Could you check a few things on this model? Use its own coordinates, in mm. Face numbers are marked on the shaded views. Round coordinates to 2 decimals unless told otherwise and drop trailing zeros. Order: outer loops, then holes, each group sorted by start corner. A loop starts at its lowest first (then second) coordinate and runs counter-clockwise, first axis right, second up.
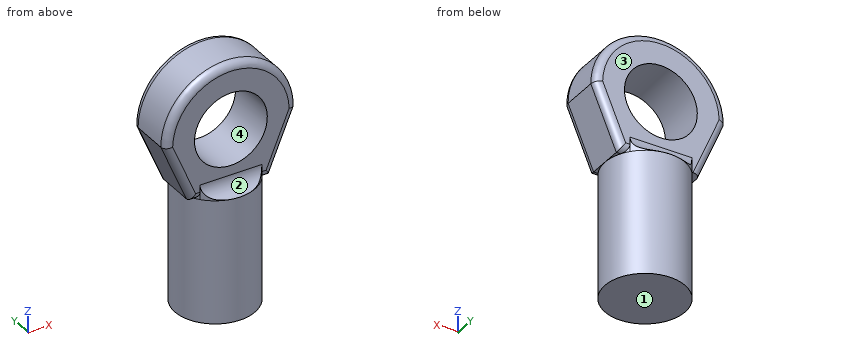
```python
from build123d import *

# Parameters (mm, degrees)
EXTRUDE_1_DEPTH     = 3.5
SKETCH_2_R          = 2.75
EXTRUDE_2_DEPTH     = 8.5
FILLET_1_R          = 1
FILLET_2_R          = 1
SKETCH_3_R          = 2.5
CUT_EXTRUDE_1_DEPTH = 15.156827953
FILLET_3_R          = 0.5


with BuildPart() as part:
    # ｽｹｯﾁ1 → ﾎﾞｽ - 押し出し1 (new body)
    with BuildSketch(Plane(origin=(0, 0, 0), x_dir=(1, 0, 0), z_dir=(0, 1, 0))):
        Polygon((-4.5, 0), (0, 0), (0, 4.145780988), (-2.75, 4.145780988), align=None)
        with BuildLine():
            Line((4.5, 0), (0, 0))
            Line((0, 0), (-4.5, 0))
            ThreePointArc((-4.5, 0), (0, -4.5), (4.5, 0))
        make_face()
        Polygon((2.75, 4.145780988), (4.5, 0), (0, 0), (0, 4.145780988), align=None)
    extrude(amount=EXTRUDE_1_DEPTH)

    # ｽｹｯﾁ2 → ﾎﾞｽ - 押し出し2 (add)
    with BuildSketch(Plane(origin=(0, 0, -4.145780988), x_dir=(-1, 0, 0), z_dir=(0, 0, -1))):
        with Locations((0, 1.75)):
            Circle(SKETCH_2_R)
    extrude(amount=EXTRUDE_2_DEPTH)

    # ﾌｨﾚｯﾄ1
    # the kernel refuses this fillet: 1 mm, written as the material it adds along each edge
    with BuildSketch(Plane(origin=(4.621320344, 0, -4.145780988), x_dir=(0, 0, 1), z_dir=(-1, 0, 0))) as fillet_1_piece_1_section:
        with BuildLine():
            CenterArc((FILLET_1_R, -FILLET_1_R), FILLET_1_R, 90, 90)
            Line((0, -FILLET_1_R), (0, 0))
            Line((0, 0), (FILLET_1_R, 0))
        make_face()
    fillet_1_piece_1 = extrude(amount=9.242640687, mode=Mode.PRIVATE)
    fillet_1_piece_1 = fillet_1_piece_1 & Plane(origin=(0, 1.75, -3.914317748), x_dir=(-1, 0, 0), z_dir=(0, 0, 1)) * Cylinder(2.75, 23, mode=Mode.PRIVATE)
    add(fillet_1_piece_1)

    # ﾌｨﾚｯﾄ2
    # the kernel refuses this fillet: 1 mm, written as the material it adds along each edge
    with BuildSketch(Plane(origin=(-4.621320344, 3.5, -4.145780988), x_dir=(0, 1, 0), z_dir=(1, 0, 0))) as fillet_2_piece_1_section:
        with BuildLine():
            CenterArc((FILLET_2_R, FILLET_2_R), FILLET_2_R, 180, 90)
            Line((0, FILLET_2_R), (0, 0))
            Line((0, 0), (FILLET_2_R, 0))
        make_face()
    fillet_2_piece_1 = extrude(amount=9.242640687, mode=Mode.PRIVATE)
    fillet_2_piece_1 = fillet_2_piece_1 & Plane(origin=(0, 1.75, -3.91431771), x_dir=(-1, 0, 0), z_dir=(0, 0, 1)) * Cylinder(2.75, 23, mode=Mode.PRIVATE)
    add(fillet_2_piece_1)

    # ｽｹｯﾁ3 → ｶｯﾄ - 押し出し1 (cut, through all)
    with BuildSketch(Plane(origin=(0, 3.5, 0), x_dir=(1, 0, 0), z_dir=(0, 1, 0))):
        with Locations(Location((0, 0, 0), (0, 0, 270))):
            Circle(SKETCH_3_R)
    extrude(amount=-CUT_EXTRUDE_1_DEPTH, mode=Mode.SUBTRACT)

    # ﾌｨﾚｯﾄ3
    # the kernel refuses this fillet: 0.5 mm, written as the material it takes off along each edge
    with BuildSketch(Plane(origin=(-0.871320344, 0, -4.145780988), x_dir=(0, 1, 0), z_dir=(-1, 0, 0))) as fillet_3_piece_1_section:
        with BuildLine():
            CenterArc((FILLET_3_R, -FILLET_3_R), FILLET_3_R, 90, 90)
            Line((0, -FILLET_3_R), (0, 0))
            Line((0, 0), (FILLET_3_R, 0))
        make_face()
    fillet_3_piece_1 = extrude(amount=3.128679656, mode=Mode.PRIVATE)
    fillet_3_piece_1 = fillet_3_piece_1 - Plane(origin=(0, 1.75, -4.02149164), x_dir=(-1, 0, 0), z_dir=(0, 0, 1)) * Cylinder(2.75, 9, mode=Mode.PRIVATE)
    add(fillet_3_piece_1, mode=Mode.SUBTRACT)
    with BuildSketch(Plane(origin=(-2.263888889, 0, -5.297386818), x_dir=(0, 1, 0), z_dir=(-0.3888888888844502, 0, 0.9212846639894848))) as fillet_3_piece_2_section:
        with BuildLine():
            CenterArc((FILLET_3_R, -FILLET_3_R), FILLET_3_R, 90, 90)
            Line((0, -FILLET_3_R), (0, 0))
            Line((0, 0), (FILLET_3_R, 0))
        make_face()
    fillet_3_piece_2 = extrude(amount=7, mode=Mode.PRIVATE)
    fillet_3_piece_2 = split(fillet_3_piece_2, bisect_by=Plane(origin=(-2.809521529, 0.121561121, -4.145780988), z_dir=(0, 0, 1)), keep=Keep.TOP, mode=Mode.PRIVATE)
    add(fillet_3_piece_2, mode=Mode.SUBTRACT)
    with BuildSketch(Plane(origin=(0, 0, 0), x_dir=(-0.9615445935244931, 0, -0.2746488570225942), z_dir=(0.2746488570225942, 0, -0.9615445935244931))) as fillet_3_piece_3:
        with BuildLine():
            CenterArc((4.5 - FILLET_3_R, FILLET_3_R), FILLET_3_R, 270, 90)
            Line((4.5 - FILLET_3_R, 0), (4.5, 0))
            Line((4.5, 0), (4.5, FILLET_3_R))
        make_face()
    revolve(axis=Axis((0, 0, 0), (0, 1, 0)), revolution_arc=211.882178867, mode=Mode.SUBTRACT)
    with BuildSketch(Plane(origin=(2.263888889, 0, -5.297386818), x_dir=(0, 1, 0), z_dir=(0.3888888888844502, 0, 0.9212846639894848))) as fillet_3_piece_4_section:
        with BuildLine():
            CenterArc((FILLET_3_R, FILLET_3_R), FILLET_3_R, 180, 90)
            Line((0, FILLET_3_R), (0, 0))
            Line((0, 0), (FILLET_3_R, 0))
        make_face()
    fillet_3_piece_4 = extrude(amount=7, mode=Mode.PRIVATE)
    fillet_3_piece_4 = split(fillet_3_piece_4, bisect_by=Plane(origin=(2.809522327, 0.121559787, -4.145780988), z_dir=(0, 0, 1)), keep=Keep.TOP, mode=Mode.PRIVATE)
    add(fillet_3_piece_4, mode=Mode.SUBTRACT)
    with BuildSketch(Plane(origin=(4, 0, -4.145780988), x_dir=(0, 1, 0), z_dir=(-1, 0, 0))) as fillet_3_piece_5_section:
        with BuildLine():
            CenterArc((FILLET_3_R, -FILLET_3_R), FILLET_3_R, 90, 90)
            Line((0, -FILLET_3_R), (0, 0))
            Line((0, 0), (FILLET_3_R, 0))
        make_face()
    fillet_3_piece_5 = extrude(amount=3.128679656, mode=Mode.PRIVATE)
    fillet_3_piece_5 = fillet_3_piece_5 - Plane(origin=(0, 1.75, -4.021491718), x_dir=(-1, 0, 0), z_dir=(0, 0, 1)) * Cylinder(2.75, 9, mode=Mode.PRIVATE)
    add(fillet_3_piece_5, mode=Mode.SUBTRACT)
    with BuildSketch(Plane(origin=(0.871320344, 3.5, -4.145780988), x_dir=(0, 0, 1), z_dir=(1, 0, 0))) as fillet_3_piece_6_section:
        with BuildLine():
            CenterArc((FILLET_3_R, FILLET_3_R), FILLET_3_R, 180, 90)
            Line((0, FILLET_3_R), (0, 0))
            Line((0, 0), (FILLET_3_R, 0))
        make_face()
    fillet_3_piece_6 = extrude(amount=3.128679656, mode=Mode.PRIVATE)
    fillet_3_piece_6 = fillet_3_piece_6 - Plane(origin=(0, 1.75, -4.021491695), x_dir=(-1, 0, 0), z_dir=(0, 0, 1)) * Cylinder(2.75, 9, mode=Mode.PRIVATE)
    add(fillet_3_piece_6, mode=Mode.SUBTRACT)
    with BuildSketch(Plane(origin=(-2.263888889, 3.5, -5.297386818), x_dir=(0.9212846639894847, 0, 0.38888888888445017), z_dir=(-0.3888888888844502, 0, 0.9212846639894848))) as fillet_3_piece_7_section:
        with BuildLine():
            CenterArc((FILLET_3_R, -FILLET_3_R), FILLET_3_R, 90, 90)
            Line((0, -FILLET_3_R), (0, 0))
            Line((0, 0), (FILLET_3_R, 0))
        make_face()
    fillet_3_piece_7 = extrude(amount=7, mode=Mode.PRIVATE)
    fillet_3_piece_7 = split(fillet_3_piece_7, bisect_by=Plane(origin=(-2.809521492, 3.378439196, -4.145780988), z_dir=(0, 0, 1)), keep=Keep.TOP, mode=Mode.PRIVATE)
    add(fillet_3_piece_7, mode=Mode.SUBTRACT)
    with BuildSketch(Plane(origin=(0, 3.5, 0), x_dir=(-0.9615445935244931, 0, -0.2746488570225942), z_dir=(0.2746488570225942, 0, -0.9615445935244931))) as fillet_3_piece_8:
        with BuildLine():
            CenterArc((4.5 - FILLET_3_R, -FILLET_3_R), FILLET_3_R, 0, 90)
            Line((4.5, -FILLET_3_R), (4.5, 0))
            Line((4.5, 0), (4.5 - FILLET_3_R, 0))
        make_face()
    revolve(axis=Axis((0, 3.5, 0), (0, 1, 0)), revolution_arc=211.882178867, mode=Mode.SUBTRACT)
    with BuildSketch(Plane(origin=(2.263888889, 3.5, -5.297386818), x_dir=(-0.9212846639894847, 0, 0.38888888888445017), z_dir=(0.3888888888844502, 0, 0.9212846639894848))) as fillet_3_piece_9_section:
        with BuildLine():
            CenterArc((FILLET_3_R, FILLET_3_R), FILLET_3_R, 180, 90)
            Line((0, FILLET_3_R), (0, 0))
            Line((0, 0), (FILLET_3_R, 0))
        make_face()
    fillet_3_piece_9 = extrude(amount=7, mode=Mode.PRIVATE)
    fillet_3_piece_9 = split(fillet_3_piece_9, bisect_by=Plane(origin=(2.80952229, 3.37844053, -4.145780988), z_dir=(0, 0, 1)), keep=Keep.TOP, mode=Mode.PRIVATE)
    add(fillet_3_piece_9, mode=Mode.SUBTRACT)


solid = part.part
```
Q1. We'd pull the mould along Z, two halves only. Please class the marked faces 1, 2, 3 and 4: released by +Z, released by -Z, zero draft, split by the parting line, or undercut.
Q2. Imagine slicing it at C-C, the plane y = 3.9. Please give me the cut outline in (x, z).
Q3. I need wall thicknesses on L1, parallel to Y at x = -3.5, z = -1; L2, parallel to X at y = 0.2, z = -1.5; L3, parallel to X at y = 1.8, z = -9.5. Which ranges of each line are inside material? Lowest first, please.
Q4. Imagine slicing it at B-B, the plane z = -9.5. Please give me the cut outline in (x, y), then the cut area to 3 significant figures.
Q5. For P1, Ø1, axis at y = 0, z = -9, coming from the +X side; P2, Ø3, axis at x = 0, z = 0, coming from the +Y side; P3, Ø3, axis at x = 3, z = -4.5, coming from the -Y side; P4, Ø1.5, axis at y = 0, z = -2, coming from the +X side, each with a flat end and sliding along its axis, tell me the tip position at first contact or that it passes through.
Filled in:
1. face 1: released by -Z
1. face 2: released by +Z
1. face 3: zero draft
1. face 4: undercut
2. outline: (-1.71, -12.65) - (1.71, -12.65) - (1.71, -3.95) - (-1.71, -3.95) - close
3. L1: y = 0 to 3.5
3. L2: x = -3.76 to -2, 2 to 3.76
3. L3: x = -2.75 to 2.75
4. outline: circle Ø5.5 at (0, 1.75)
4. area: 23.8 mm2
5. P1: stops at x = 2.45
5. P2: passes through
5. P3: stops at y = -0.55
5. P4: stops at x = 3.91
